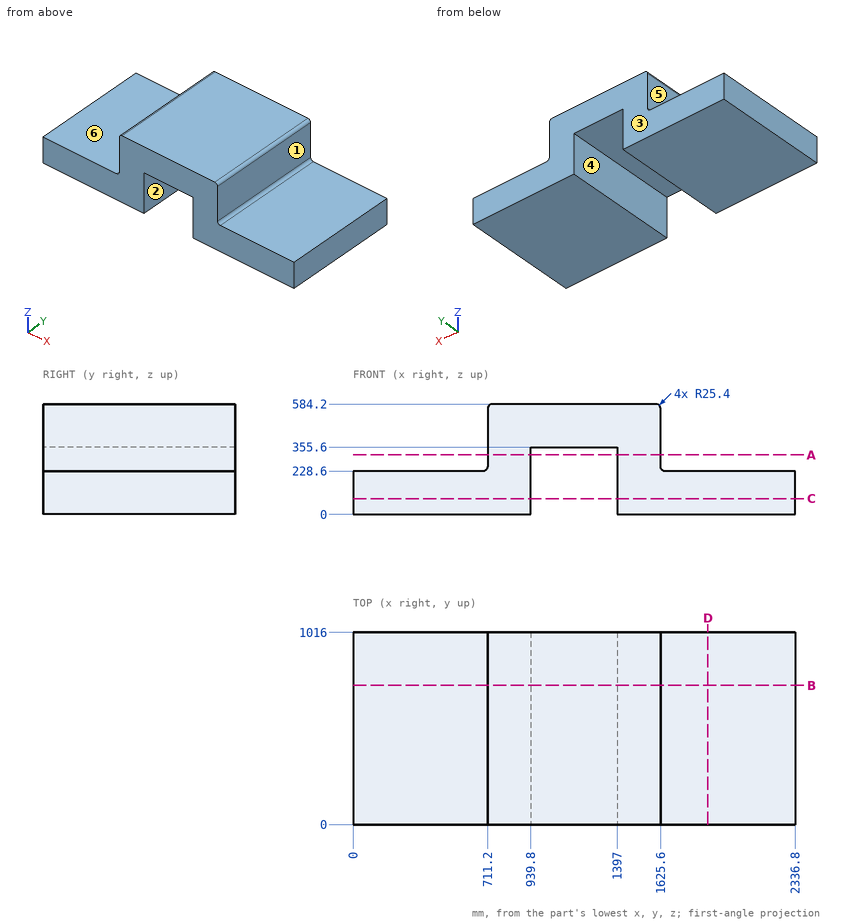
Print and shaded views of the part. All mm, measured from the part's lowest x, y and z. A direction names the side the tool comes from. Give positions to 0.01 mm unless a question says otherwise; leave off trailing zeros. Loops run counter-clockwise (first coordinate to the right, second up) from the corner with the lowest first, then second, coordinate; pieces in that order, holes last. Notation, with made-up numbers: (-13.5, 55.25) -> (37.5, 55.25) arc R30 ccw to (37.5, 77.25) -> close; hole circle Ø10 at (-1, 41). An arc over 180 degrees is marked (long way). Use a Markdown table: item, result.
1. Flat gauge pins, fed straight in: pin 1 (4 mm diameter, centred on y = 869.5, z = 472.5, fed in from -X); pin 2 (8 mm diameter, centred on y = 299, z = 521.5, fed in from +X). Where does each tip first touch, or does it go through?
Check result:
| item | result |
|---|---|
| pin 1 | stops at x = 711.2 |
| pin 2 | stops at x = 1625.6 |
2. Slice it at B-B (y = 736). List the corners of the cut face in (x, z), plus the area to 3 significant figures.
Check result:
| item | result |
|---|---|
| outline | (0, 0) -> (939.8, 0) -> (939.8, 355.6) -> (1397, 355.6) -> (1397, 0) -> (2336.8, 0) -> (2336.8, 228.6) -> (1651, 228.6) arc R25.4 cw to (1625.6, 254) -> (1625.6, 558.8) arc R25.4 ccw to (1600.2, 584.2) -> (736.6, 584.2) arc R25.4 ccw to (711.2, 558.8) -> (711.2, 254) arc R25.4 cw to (685.8, 228.6) -> (0, 228.6) -> close |
| area | 697,000 mm^2 |
3. Wall check: L1, parallel to X at y = 298.5, z = 331; L2, parallel to X at y = 105.5, z = 145.5; L3, parallel to Z at x = 451.5, y = 776.5. Give the ranges that are in metal, low to high. Write a range as [from, to].
Check result:
| item | result |
|---|---|
| L1 | x = [711.2, 939.8], [1397, 1625.6] |
| L2 | x = [0, 939.8], [1397, 2336.8] |
| L3 | z = [0, 228.6] |
4. Mould opens along X. For the marked faces 4, 5 and 6 say: pulls with the +X half, pulls with the -X half, needs draft (parallel to the pull), parting line crosses it, or undercut.
Check result:
| item | result |
|---|---|
| face 4 | undercut |
| face 5 | pulls with the -X half |
| face 6 | needs draft |
5. Slice it at A-A (z = 315). List the corners of the cut face in (x, y), plus the area to 3 significant figures.
Check result:
| item | result |
|---|---|
| outline | (711.2, 0) -> (939.8, 0) -> (939.8, 1016) -> (711.2, 1016) -> close; (1397, 0) -> (1625.6, 0) -> (1625.6, 1016) -> (1397, 1016) -> close |
| area | 465,000 mm^2 |
6. Slice it at D-D (x = 1875.5). List the corners of the cut face in (y, z), plus the area to 3 significant figures.
Check result:
| item | result |
|---|---|
| outline | (0, 0) -> (1016, 0) -> (1016, 228.6) -> (0, 228.6) -> close |
| area | 232,000 mm^2 |
7. Which spindle directions (+Z, -Z, +X, -X, +Y, -Y) get a long thin tool onto all of the face, cutting with end or side? Do the marked faces 1, 2 and 3. Say none if no direction does.
Check result:
| item | result |
|---|---|
| face 1 | +Z, +X, +Y, -Y |
| face 2 | -Z, +Y, -Y |
| face 3 | +Z, -Z, +X, -X, +Y |
8. Slice it at C-C (z = 84). List the corners of the cut face in (x, y), plus the area to 3 significant figures.
Check result:
| item | result |
|---|---|
| outline | (0, 0) -> (939.8, 0) -> (939.8, 1016) -> (0, 1016) -> close; (1397, 0) -> (2336.8, 0) -> (2336.8, 1016) -> (1397, 1016) -> close |
| area | 1,910,000 mm^2 |
